For this review, take the finished solid that the model builds, in its own axes (mm). A direction names the side the tool comes from. Coordinates: 2 decimals unless noted, no trailing zeros. Write each loop counter-clockwise with the first axis right and the second up, starting at its lowest first coordinate (ties: lowest second). Pieces come first, ordered by that corner, then holes. Notation, with made-up numbers: M 36,47.5 L 93,47.5 A19 ccw 93,72.5 Z; hole C 44,29 d6. An arc over 180 degrees is marked long. One line per question, with ' | ' between items.
from build123d import *

# Parameters (mm, degrees)
SKETCH_1_R      = 2.5
EXTRUDE_1_DEPTH = 2
SKETCH_2_R      = 2
EXTRUDE_3_DEPTH = 2
EXTRUDE_4_REACH = 91.774
SKETCH_4_R      = 4


with BuildPart() as part:
    # Sketch 1 → Extrude 1 (new body)
    with BuildSketch(Plane(origin=(0, 0, 0), x_dir=(1, 0, 0), z_dir=(0, 1, 0))):
        Polygon((10.502525317, -60), (60, -10.502525317), (60, 0), (20, 0), (20, -20), (0, -20), (0, -60), align=None)
        with Locations(Location((10, -52, 0), (0, 0, 270))):
            Circle(SKETCH_1_R, mode=Mode.SUBTRACT)
        with Locations(Location((52, -10, 0), (0, 0, 270))):
            Circle(SKETCH_1_R, mode=Mode.SUBTRACT)
    extrude(amount=EXTRUDE_1_DEPTH)



with BuildPart() as body_2:
    # Sketch 2 → Extrude 3 (new body)
    with BuildSketch(Plane(origin=(23.112372436, 18.871173071, 23.112372436), x_dir=(-0.7071067811865475, 0, 0.7071067811865477), z_dir=(0.6123724356957955, 0.4999999999999981, 0.6123724356957954))):
        Polygon((-3, 16.786030205), (-15, 16.786030205), (-15, -13.213969795), (15, -13.213969795), (15, 11.786030205), (-3, 11.786030205), align=None)
        with Locations(Location((-12, -10.713969795, 0), (0, 0, 180))):
            Circle(SKETCH_2_R, mode=Mode.SUBTRACT)
        with Locations(Location((12, -10.713969795, 0), (0, 0, 180))):
            Circle(SKETCH_2_R, mode=Mode.SUBTRACT)
        with Locations(Location((-12, 14.286030205, 0), (0, 0, 180))):
            Circle(SKETCH_2_R, mode=Mode.SUBTRACT)
    extrude(amount=EXTRUDE_3_DEPTH)


with BuildPart() as part_1:
    add(part.part)

    add(body_2.part)  # Extrude 4 merges body 2
    # Extrude 4: up to this plane
    extrude_4_end = Plane(origin=(23.112372436, 18.871173071, 23.112372436), z_dir=(0.6123724356957954, 0.4999999999999981, 0.6123724356957952))
    # Sketch 4 → Extrude 4 (add, up to the surface)
    with BuildSketch(Plane(origin=(0, 2, 0), x_dir=(1, 0, 0), z_dir=(0, 1, 0)), mode=Mode.PRIVATE) as extrude_4_sk1:
        with Locations(Location((25.511596423, -18.440528611, 0), (0, 0, 315))):
            Circle(SKETCH_4_R)
    extrude_4_tool1 = split(extrude(extrude_4_sk1.sketch, amount=EXTRUDE_4_REACH, mode=Mode.PRIVATE), bisect_by=extrude_4_end, keep=Keep.BOTH, mode=Mode.PRIVATE)
    add(extrude_4_tool1.solids().sort_by_distance((25.511596, 2, 18.440529))[0])


solid = part_1.part
1. Take a section at C-C on y = 22. State the section outline as (x, z) points, plus the area to 3 significant figures.
Computed values:
outline: M 11.23,32.44 L 22.55,21.12 A4 ccw 28.2,15.47 L 32.44,11.23 L 34.07,12.86 L 12.86,34.07 Z | area: 92.8 mm2
2. Draft analysis for pull direction Y (two halves, no side actions). For faces 6 (the flat face through (30.876, 7.022, 26.633)), 7 (the flat face through (25.191, 18.143, 24.894)), 8 (the flat face through (23, 0, 23)), 9 (the flat face through (5, 1, 60)), state which applies: pulls with the +Y half, pulls with the -Y half, needs draft (parallel to the pull), parting line crosses it, or undercut.
Computed values:
face 6: undercut | face 7: pulls with the +Y half | face 8: pulls with the -Y half | face 9: needs draft
3. Take a section at D-D on x = 4.5. State the section outline as (y, z) points, plus the area to 3 significant figures.
Computed values:
outline: M 0,20 L 2,20 L 2,60 L 0,60 Z | area: 80.0 mm2
4. For line 1 along X through (y, z) = (1.6, 10); line 2 along Y through (x, z) = (51.5, 3); line 3 along X through (y, z) = (9, 26), list the stretches that pass through material, from the lowest coordinate up.
Computed values:
line 1: x = 20 to 49.5, 54.5 to 60 | line 2: y = 0 to 2 | line 3: x = 28.28 to 29.38, 30.24 to 31.55
5. Clearance check with flat-ended pins moving along their axes: P1, Ø6, axis at y = 15.5, z = 28.5, coming from the -X side; P2, Ø4, axis at x = 23, z = 44.5, coming from the +Y side; P3, Ø5, axis at y = 17.5, z = 26, coming from the -X side; P4, Ø5, axis at x = 25, z = 32, coming from the -Y side. State where each tip first meets the part, or that it passes through.
Computed values:
P1: stops at x = 16.6 | P2: stops at y = 2 | P3: stops at x = 18.12 | P4: stops at y = 0
6. Take a section at A-A on z = 52. State the section outline as (x, y) points.
Computed values:
outline: M 0,0 L 7.5,0 L 7.5,2 L 0,2 Z; M 12.5,0 L 18.5,0 L 18.5,2 L 12.5,2 Z
7. Machinability: for faces 1 (the flat face through (12.795, 20.134, 34.008)), 2 (the flat face through (0, 1, 40)), 3 (the flat face through (35.028, 17.636, 13.815)), 4 (the flat face through (35.96, 4.83, 23.35)), 5 (the flat face through (23.97, 17.14, 23.67)), which of the approach directions +Z, -Z, +X, -X, +Y, -Y give a long, thin tool a straight path to every point of the face, cutting with its end or side? Answer none if there is none.
Computed values:
face 1: +Z, -X, +Y | face 2: +Z, -Z, -X, +Y, -Y | face 3: -Z, +X, +Y | face 4: +Z, +X | face 5: none
8. Take a section at B-B on x = 34. State the section outline as (y, z) points, plus the area to 3 significant figures.
Computed values:
outline: M 0,0 L 2,0 L 2,36.5 L 0,36.5 Z; M 4.33,24.09 L 18.18,12.79 L 22.18,12.79 L 5.33,26.54 Z | area: 123 mm2
